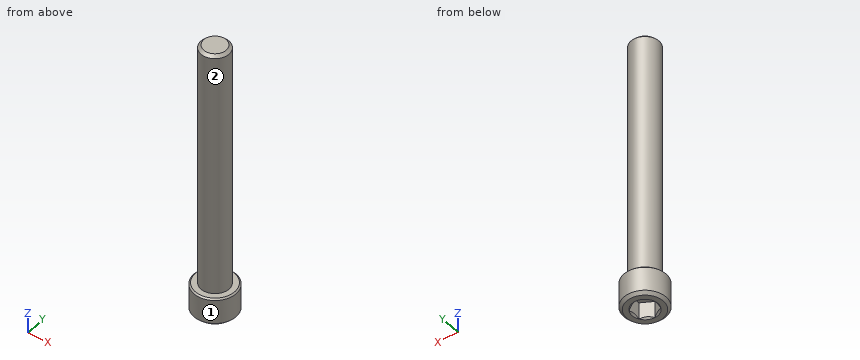
```python
from build123d import *

# Parameters (mm, degrees)
SKETCH1_R          = 3.96875
EXTRUDE1_DEPTH     = 69.85
CHAMFER3_SIZE      = 0.79375
SKETCH6_R          = 5.953125
EXTRUDE2_DEPTH     = 7.9375
CUT_EXTRUDE1_DEPTH = 4.7625
SKETCH8_R          = 3.666174209
CUT_EXTRUDE2_DEPTH = 0.79375
CUT_EXTRUDE2_DRAFT = -45
CHAMFER1_SIZE      = 0.79375
CHAMFER2_SIZE      = 0.396875


with BuildPart() as part:
    # Sketch1 → Extrude1 (new body)
    with BuildSketch(Plane.XY):
        Circle(SKETCH1_R)
    extrude(amount=-EXTRUDE1_DEPTH)

    # Chamfer3
    chamfer3_edges = [part.edges().sort_by_distance(p)[0] for p in [
        (-3.96875, 0, 0),
    ]]
    chamfer(chamfer3_edges, length=CHAMFER3_SIZE)

    # Sketch5 → partially thread (revolve)
    with BuildSketch(Plane(origin=(0, 0, 0), x_dir=(0, 0, -1), z_dir=(1, 0, 0))):
        Polygon((69.85, 3.96875), (28.575, 3.96875), (24.60625, 0), (28.575, 0), (69.85, 0), align=None)
    revolve(axis=Axis((0, 0, 0), (0, 0, -1)))

    # Sketch6 → Extrude2 (add)
    with BuildSketch(Plane(origin=(0, 0, -69.85), x_dir=(-1, 0, 0), z_dir=(0, 0, -1))):
        Circle(SKETCH6_R)
    extrude(amount=EXTRUDE2_DEPTH)

    # Sketch7 → Cut-Extrude1 (cut)
    with BuildSketch(Plane(origin=(0, 0, -77.7875), x_dir=(-1, 0, 0), z_dir=(0, 0, -1))):
        Polygon((0, 3.666174209), (-3.175, 1.833087105), (-3.175, -1.833087105), (0, -3.666174209), (3.175, -1.833087105), (3.175, 1.833087105), align=None)
    extrude(amount=-CUT_EXTRUDE1_DEPTH, mode=Mode.SUBTRACT)


with BuildPart() as cut_extrude2_tool:
    # Sketch8 → Cut-Extrude2 (with draft: the straight prism first)
    with BuildSketch(Plane(origin=(0, 0, -77.7875), x_dir=(-1, 0, 0), z_dir=(0, 0, -1))):
        Circle(SKETCH8_R)
    extrude(amount=-CUT_EXTRUDE2_DEPTH)
    # Cut-Extrude2: the draft: its side faces are tilted about the plane it starts from
    cut_extrude2_sides = [cut_extrude2_tool.faces().sort_by_distance(p)[0] for p in [
        (3.666174209, 0, -77.390625),
    ]]
    draft(cut_extrude2_sides, Plane(origin=(0, 0, -77.7875), x_dir=(-1, 0, 0), z_dir=(0, 0, -1)), CUT_EXTRUDE2_DRAFT)


with BuildPart() as part_1:
    add(part.part)

    # Cut-Extrude2: cut by cut_extrude2_tool
    add(cut_extrude2_tool.part, mode=Mode.SUBTRACT)

    # Chamfer1
    chamfer1_edges = [part_1.edges().sort_by_distance(p)[0] for p in [
        (5.953125, 0, -77.7875),
    ]]
    chamfer(chamfer1_edges, length=CHAMFER1_SIZE)

    # Chamfer2
    chamfer2_edges = [part_1.edges().sort_by_distance(p)[0] for p in [
        (5.953125, 0, -69.85),
    ]]
    chamfer(chamfer2_edges, length=CHAMFER2_SIZE)


solid = part_1.part
```
Here's how the part is built. I have some questions about the finished solid (model axes, mm). Face numbers are marked on the shaded views. A direction names the side the tool comes from. Round coordinates to 2 decimals unless told otherwise and drop trailing zeros. Write each loop counter-clockwise with the first axis right and the second up, starting at its lowest first coordinate (ties: lowest second). Pieces come first, ordered by that corner, then holes. Notation, with made-up numbers: M 57.25,2 L 74.25,2 A20 cw 74.25,16 Z; hole C 60.5,84 d6. An arc over 180 degrees is marked long. Answer as CSV lines item,"result". Start each with the question number.
1. Suppose I cut it at B-B on z = -62. Write out the boundary of the cut face in (x, y).
2. I need wall thicknesses on probe 1 along Z at (x, y) = (-2, 1.75) (3 decimals); probe 2 along Z at (x, y) = (-0.5, -5); probe 3 along Y at (x, z) = (1.5, -50). Which ranges of each line are inside material? Lowest first, please.
3. I'm going to push flat-ended pins straight in: pin 1 Ø6 at (x, y) = (-1.5, 2.5) entering from -Z; pin 2 Ø1.5 at (x, z) = (2, -21) entering from +Y; pin 3 Ø4 at (x, z) = (4.5, -55) entering from +Y; pin 4 Ø1.5 at (x, y) = (-2.5, -1) entering from -Z. Where does each tip first touch, or does it pass through?
4. On a 3-axis mill with a long thin cutter (end or side, diameter ignored), from which of +Z, -Z, +X, -X, +Y, -Y can I reach the whole of each face in a straight line? I mean the marked faces 1 and 2. Say none if no direction works.
Check result:
1,outline,"C 0,0 d7.94"
2,probe 1,"z = -73.025 to 0"
2,probe 2,"z = -77.79 to -69.85"
2,probe 3,"y = -3.67 to 3.67"
3,pin 1,"stops at z = -77.79"
3,pin 2,"stops at y = 3.77"
3,pin 3,"stops at y = 3.08"
3,pin 4,"stops at z = -77.56"
4,face 1,"+Z, -Z"
4,face 2,"+Z"
